Can you work these out from the model? Positions are in its coordinate system, mm. Give positions to 0.01 mm unless a question says otherwise; leave off trailing zeros. Write each question's results on one line, items separated by ' | '. Start each with the question number.
from build123d import *

# Parameters (mm, degrees)
SKETCH1_W           = 45
SKETCH1_H           = 200
BOSS_EXTRUDE1_DEPTH = 2
SKETCH2_R           = 2
CUT_EXTRUDE1_DEPTH  = 103.519510338
SKETCH5_W           = 45
SKETCH5_H           = 2
BOSS_EXTRUDE3_DEPTH = 50
SKETCH6_R           = 2
CUT_EXTRUDE3_DEPTH  = 50


with BuildPart() as part:
    # Sketch1 → Boss-Extrude1 (new body)
    with BuildSketch(Plane.XY):
        Rectangle(SKETCH1_W, SKETCH1_H)
    extrude(amount=BOSS_EXTRUDE1_DEPTH)

    # Sketch2 → Cut-Extrude1 (cut, through all)
    with BuildSketch(Plane.XY.offset(2)):
        with Locations((2.5, -70)):
            Circle(SKETCH2_R)
        with Locations((2.5, 70)):
            Circle(SKETCH2_R)
    extrude(amount=-CUT_EXTRUDE1_DEPTH, mode=Mode.SUBTRACT)

    # Sketch5 → Boss-Extrude3 (add)
    with BuildSketch(Plane.XZ.offset(100)):
        with Locations((0, 1)):
            Rectangle(SKETCH5_W, SKETCH5_H)
    extrude(amount=BOSS_EXTRUDE3_DEPTH)

    # Sketch6 → Cut-Extrude3 (cut)
    with BuildSketch(Plane(origin=(0, 0, 0), x_dir=(-1, 0, 0), z_dir=(0, 0, -1))):
        with Locations((-2.5, -120)):
            Circle(SKETCH6_R)
    extrude(amount=-CUT_EXTRUDE3_DEPTH, mode=Mode.SUBTRACT)


solid = part.part
Q1. If I drill on probe 1 along Y at (x, z) = (2.5, 0.85); probe 2 along Y at (x, z) = (2, 1.55), over which ranges is the centre line in solid material (lowest first)? Write a range as from..to.
Q2. Thinking about a two-plate mould opening in X: for faces 1 (the cylindrical face through (2.24, -68.017, 1.014)), 2 (the flat face through (0, -23, 0)), which applies, released by +X, released by -X, zero draft, split by the parting line, or undercut?
Q3. Will this pin go through, and if not, where does the flat tip stop? P1, Ø3, axis at x = 2.5, y = -120, coming from the -Z side.
Findings below:
1) probe 1: y = -150..-122, -118..-72, -68..68, 72..100 | probe 2: y = -150..-121.94, -118.06..-71.94, -68.06..68.06, 71.94..100
2) face 1: undercut | face 2: zero draft
3) P1: passes through
